Study the drawing (mm; zero at the part's minimum x, y, z) and answer. Give positions to 0.01 mm unless a question says otherwise; leave off trailing zeros. Order: outer loops, then holes, each group sorted by start corner. A loop starts at its lowest first (then second) coordinate and runs counter-clockwise, first axis right, second up. Notation, with made-up numbers: (63.25, 58) - (72.25, 58) arc R18 cw to (72.25, 82) - close; hole circle Ø4 at (34, 52.5). An arc over 180 degrees is marked (long way). Use CSV: the item, a comma, the result in double quotes.
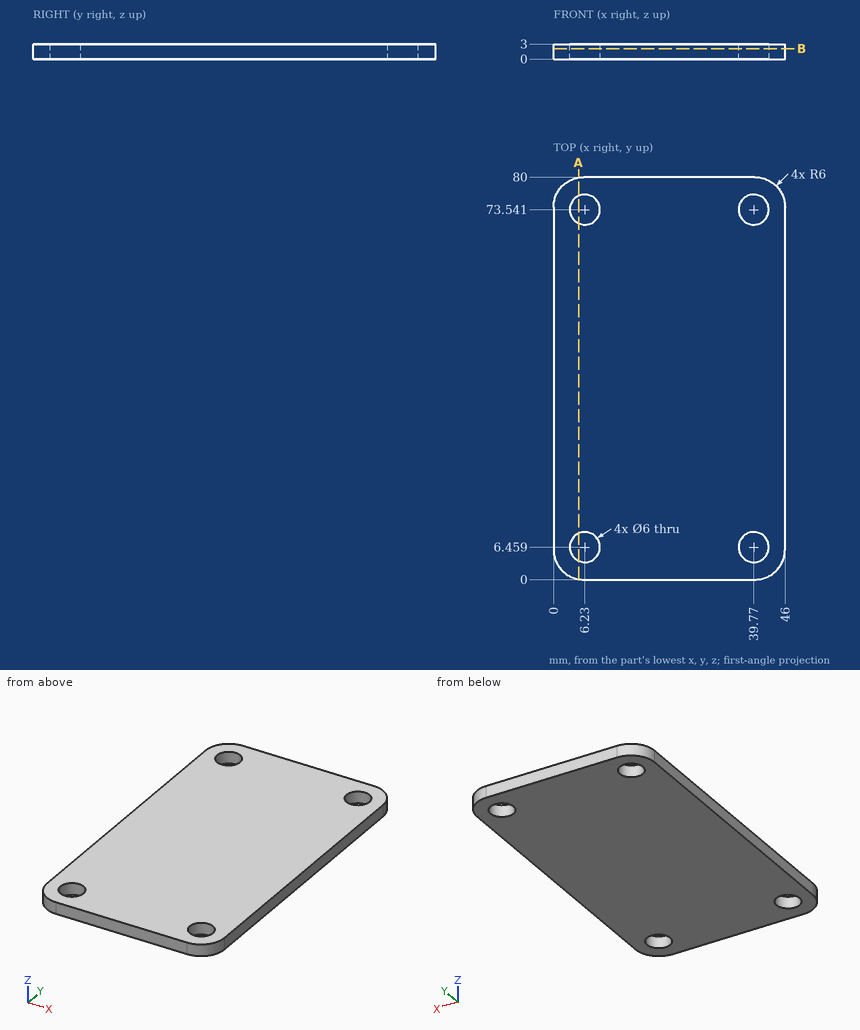
Item 1: The part is cut by section B-B (z = 2.1). Give the vertices of the cut face in (x, y).
Taken from the geometry:
outline,"(0, 6) arc R6 ccw to (6, 0) - (40, 0) arc R6 ccw to (46, 6) - (46, 74) arc R6 ccw to (40, 80) - (6, 80) arc R6 ccw to (0, 74) - close; hole circle Ø6 at (6.23, 6.46); hole circle Ø6 at (6.23, 73.54); hole circle Ø6 at (39.77, 6.46); hole circle Ø6 at (39.77, 73.54)"
Item 2: This flat-tipped pin is pushed along its axis until it touches: pin 1 (5 mm diameter, centred on x = 39.77, y = 73.54, fed in from -Z). Where does it stop, or does it pass through?
Taken from the geometry:
pin 1,"through"
Item 3: Find the intervals of material crossed by line 1 along Y through (x, z) = (7, 1.8); line 2 along Y through (x, z) = (8.5, 1.75) (1 decimal), in increasing order.
Taken from the geometry:
line 1,"0 to 3.56, 9.36 to 70.64, 76.44 to 80"
line 2,"0 to 4.5, 8.4 to 71.6, 75.5 to 80"
Item 4: The part is cut by section A-A (x = 5). Give the vertices of the cut face in (y, z) (1 decimal), and give its area (3 significant figures).
Taken from the geometry:
outline,"(0.1, 0) - (3.7, 0) - (3.7, 3) - (0.1, 3) - close; (9.2, 0) - (70.8, 0) - (70.8, 3) - (9.2, 3) - close; (76.3, 0) - (79.9, 0) - (79.9, 3) - (76.3, 3) - close"
area,"207 mm^2"
